Autodesk Inventor part; units mm, degrees
ref_plane "YZ Plane" through (0, 0, 0) normal (1, 0, 0) x (0, 1, 0)
ref_plane "XZ Plane" through (0, 0, 0) normal (0, 1, 0) x (-1, 0, 0)
ref_plane "XY Plane" through (0, 0, 0) normal (0, 0, 1) x (1, 0, 0)
sketch "Szkic1" plane through (0, 0, 0) normal (0, 0, 1) x (1, 0, 0)
  line L0 (0, 0) -> (14, 0)
  line L1 (14, 0) -> (14, 23)
  line L2 (14, 23) -> (0, 23)
  line L3 (0, 23) -> (0, 0)
  line L4 (14, 0) -> (63, 0)
  line L5 (63, 0) -> (63, 11.5)
  line L6 (63, 11.5) -> (14, 11.5)
  line L7 (14, 11.5) -> (14, 0)
  line L8 (63, 0) -> (83, 0)
  line L9 (83, 0) -> (83, 7.5)
  line L10 (83, 7.5) -> (63, 7.5)
  line L11 (63, 7.5) -> (63, 0)
  line L12 (83, 0) -> (124, 0)
  line L13 (124, 0) -> (124, 5)
  line L14 (124, 5) -> (83, 5)
  line L15 (83, 5) -> (83, 0)
  point P0 (14, 11.5)
  dimension "d0" = 14
  dimension "d1" = 23
  dimension "d2" = 49
  dimension "d3" = 11.5
  dimension "d4" = 20
  dimension "d5" = 7.5
  dimension "d6" = 41
  dimension "d7" = 5
revolve "Obrót1" add sketch "Szkic1" angle 360 mid plane about axis through (14, 0, 0) along (1, 0, 0)
sketch "Szkic2" plane through (0, 0, 0) normal (-1, 0, 0) x (0, 0, 1)
  circle A0 centre (0, 0) radius 23
hole "Otwór1" at (0, 0, 0) direction (1, 0, 0) diameter 19 depth 57 tip angle 118
chamfer "Faza1" distance 1 angle 45 1 edges at (124, 5, 0) measured on face at (124, 0.8193, 0.3214)
fillet "Zaokrąglenie powierzchni1" radius 2 1 edges at (83, 5, 0)
sketch "Szkic3" plane through (0, 0, 0) normal (1, 0, 0) x (0, 1, 0)
  circle A0 centre (0, 0) radius 23
  line L0 (23, 0) -> (15.5, 0)
  line L1 (15.5, 0) -> (3.9555, 22.6573)
  line L2 (-23, 0) -> (-15.5, 0)
  line L3 (-15.5, 0) -> (-3.9555, 22.6573)
  line L4 (-15.5, 0) -> (9.9289, 0) construction
  dimension "d20" = 7.5
  dimension "d21" = 117
  dimension "d22" = 7.5
  dimension "d23" = 63
extrude "Wyciągnięcie proste1" cut sketch "Szkic3" along normal blind 14 contours L0 L1 A0 | A0 L3 L2
sketch "Szkic4" plane through (0, 0, 0) normal (1, 0, 0) x (0, 1, 0)
  circle A0 centre (0, 14.411) radius 5
  point P0 (0, 0)
  dimension "d26" = 10
extrude "Wyciągnięcie proste2" add sketch "Szkic4" against normal blind 6
sketch "Szkic5" plane through (-6, 0, 14.411) normal (-1, 0, 0) x (0, 0, 1)
  point P0 (-14.411, 0)
  point P1 (0, 0)
hole "Otwór2" at (-6, 0, 14.411) direction (1, 0, 0) diameter 2 end through all
sketch "Szkic6" plane through (0, 0, 0) normal (0, 1, 0) x (-1, 0, 0)
  line L0 (-14, 11.5) -> (-63, 11.5)
  line L1 (-40, 7) -> (-52, 7)
  line L2 (-56, 11) -> (-56, 11.5)
  line L3 (-56, 11.5) -> (-36, 11.5)
  line L4 (-36, 11.5) -> (-36, 11)
  line L5 (0, 0) -> (0, 22.6573)
  arc A0 (-40, 7) -> (-36, 11) centre (-40, 11) ccw
  arc A1 (-56, 11) -> (-52, 7) centre (-52, 11) ccw
  dimension "d36" = 20
  dimension "d37" = 36
  dimension "d38" = 4.5
  dimension "d39" = 4
  dimension "d40" = 4
extrude "Wyciągnięcie proste3" cut sketch "Szkic6" along normal through all both and the other way through all
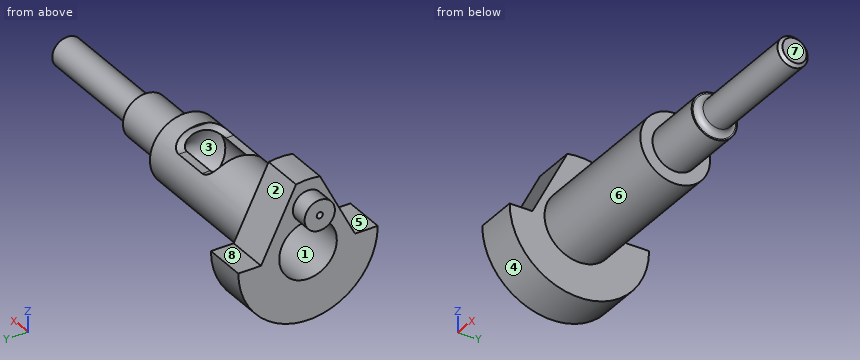
Model file for the job. Use its own axes, mm. Face numbers are marked on the shaded views. A direction names the side the tool comes from. Round coordinates to 2 decimals unless told otherwise and drop trailing zeros. Write each loop counter-clockwise with the first axis right and the second up, starting at its lowest first coordinate (ties: lowest second). Pieces come first, ordered by that corner, then holes. Notation, with made-up numbers: (88, -14) - (101, -14) arc R11 cw to (101, 5) - close; hole circle Ø8 at (39, 3.25). An arc over 180 degrees is marked (long way). Use CSV: the item, a comma, the result in double quotes. Start each with the question number.
Item 1: Band-saw the part on B-B (z = 17). Write the cut outline in (x, y), and give its area (3 significant figures).
Item 2: Drill centre lines: L1, parallel to Y at x = 27.5, z = 0; L2, parallel to X at y = 12, z = 5. Where is each one in solid material? Low to high. Write a range as [from, to].
Item 3: Band-saw the part on A-A (x = 11.5). Write the cut outline in (y, z).
Item 4: Band-saw the part on C-C (x = 24.5). Write the cut outline in (y, z), and give its area (3 significant figures).
Item 5: Pin check, flat tips, straight feed: P1, Ø3, axis at x = 95, z = 0, coming from the -Y side; P2, Ø2, axis at x = 43, y = -8, coming from the +Z side; P3, Ø2.5, axis at y = 0, z = 14.411, coming from the +X side; P4, Ø8, axis at x = 104.5, y = -10.5, coming from the -Z side. Stop position of each tip, or through.
Item 6: Band-saw the part on D-D (x = 99). Write the cut outline in (y, z), and give its area (3 significant figures).
Item 7: Tool access for the marked faces 5, 6, 7 and 8: list every direction of +Z, -Z, +X, -X, +Y, -Y with a clear straight run to the whole face (end or side of a thin tool).
Item 8: Two-plate mould, pull along Y, no slides. Class the marked faces 1, 2, 3 and 4: released by +Y, released by -Y, zero draft, split by the parting line, or undercut.
Checked values:
1,outline,"(-6, -4.28) - (0, -4.28) - (0, -6.84) - (14, -6.84) - (14, 6.84) - (0, 6.84) - (0, 4.28) - (-6, 4.28) - close"
1,area,"243 mm²"
2,L1,"y = [-11.5, -9.5], [9.5, 11.5]"
2,L2,"x = [0, 14]"
3,outline,"(-23, 0) arc R23 ccw to (23, 0) - (15.5, 0) - (3.96, 22.66) arc R23 ccw to (-3.96, 22.66) - (-15.5, 0) - close; hole circle Ø19 at (0, 0); hole circle Ø2 at (0, 14.41)"
4,outline,"circle Ø23 at (0, 0); hole circle Ø19 at (0, 0)"
4,area,"132 mm²"
5,P1,"stops at y = -5"
5,P2,"stops at z = 7"
5,P3,"stops at x = 14"
5,P4,"passes through"
6,outline,"circle Ø10 at (0, 0)"
6,area,"78.5 mm²"
7,face 5,"+Z, +X, -X, -Y"
7,face 6,"+X"
7,face 7,"+Z, -Z, +X, +Y, -Y"
7,face 8,"+Z, +X, -X, +Y"
8,face 1,"undercut"
8,face 2,"released by +Y"
8,face 3,"undercut"
8,face 4,"split by the parting line"
